Verification items for the finished model (mm, model axes). A direction names the side the tool comes from. Coordinates: 2 decimals unless noted, no trailing zeros. Order: outer loops, then holes, each group sorted by start corner. A loop starts at its lowest first (then second) coordinate and runs counter-clockwise, first axis right, second up. Notation, with made-up numbers: (-16.75, 11.25) -> (-5.75, 11.25) arc R20 cw to (-5.75, 37.25) -> close; hole circle Ø8 at (54.5, -6.75). An arc over 180 degrees is marked (long way). Answer as CSV lines item,"result".
```python
from build123d import *

# Parameters (mm, degrees)
SKETCH1_R           = 62.5
SKETCH1_R_2         = 22.5
BOSS_EXTRUDE1_DEPTH = 75
BOSS_EXTRUDE2_DEPTH = 25
SKETCH4_W           = 250
SKETCH4_H           = 270
BOSS_EXTRUDE3_DEPTH = 40
RIB5_REACH          = 417.482
SKETCH6_WALL_W      = 1103.483628374
SKETCH6_WALL_H      = 25
SKETCH9_R           = 6.25
SKETCH9_R_2         = 12.5
CUT_EXTRUDE4_DEPTH  = 40


with BuildPart() as part:
    # Sketch1 → Boss-Extrude1 (new body)
    with BuildSketch(Plane.XY):
        Circle(SKETCH1_R)
        Circle(SKETCH1_R_2, mode=Mode.SUBTRACT)
    extrude(amount=BOSS_EXTRUDE1_DEPTH)

    # Sketch3 → Boss-Extrude2 (add)
    with BuildSketch(Plane(origin=(0, 0, 0), x_dir=(-1, 0, 0), z_dir=(0, 0, -1))):
        with BuildLine():
            Line((-62.5, 0), (-125, -250))
            Line((-125, -250), (125, -250))
            Line((125, -250), (62.5, 0))
            ThreePointArc((62.5, 0), (0, -62.5), (-62.5, 0))
        make_face()
    extrude(amount=-BOSS_EXTRUDE2_DEPTH)

    # Sketch4 → Boss-Extrude3 (add)
    with BuildSketch(Plane.XZ.offset(250)):
        with Locations((0, 135)):
            Rectangle(SKETCH4_W, SKETCH4_H)
    extrude(amount=BOSS_EXTRUDE3_DEPTH)

    # Sketch6 wall → Rib5 (add, up to next)
    with BuildSketch(Plane(origin=(0, -156.25, 172.5), x_dir=(0, 0.693108716252, -0.720833064902), z_dir=(0, 0.720833064902, 0.693108716252)), mode=Mode.PRIVATE) as rib5_sk1:
        Rectangle(SKETCH6_WALL_W, SKETCH6_WALL_H)
    rib5_tool1 = extrude(rib5_sk1.sketch, amount=-RIB5_REACH, mode=Mode.PRIVATE) - part.part
    add(rib5_tool1.solids().sort_by_distance((0, -156.25, 172.5))[0])

    # Sketch9 → Cut-Extrude4 (cut)
    with BuildSketch(Plane.XZ.offset(290)):
        with Locations(Location((-110, 225, 0), (0, 0, 270))):
            Circle(SKETCH9_R)
        with Locations(Location((-110, 255, 0), (0, 0, 270))):
            Circle(SKETCH9_R)
        with Locations(Location((95, 75, 0), (0, 0, 270))):
            Circle(SKETCH9_R_2)
        with Locations(Location((-95, 240, 0), (0, 0, 270))):
            Circle(SKETCH9_R_2)
        with Locations(Location((-80, 255, 0), (0, 0, 270))):
            Circle(SKETCH9_R)
        with Locations(Location((-80, 225, 0), (0, 0, 270))):
            Circle(SKETCH9_R)
        with Locations(Location((110, 225, 0), (0, 0, 270))):
            Circle(SKETCH9_R)
        with Locations(Location((95, 240, 0), (0, 0, 270))):
            Circle(SKETCH9_R_2)
        with Locations(Location((110, 255, 0), (0, 0, 270))):
            Circle(SKETCH9_R)
        with Locations(Location((80, 255, 0), (0, 0, 270))):
            Circle(SKETCH9_R)
        with Locations(Location((80, 225, 0), (0, 0, 270))):
            Circle(SKETCH9_R)
        with Locations(Location((110, 90, 0), (0, 0, 270))):
            Circle(SKETCH9_R)
        with Locations(Location((110, 60, 0), (0, 0, 270))):
            Circle(SKETCH9_R)
        with Locations(Location((80, 60, 0), (0, 0, 270))):
            Circle(SKETCH9_R)
        with Locations(Location((80, 90, 0), (0, 0, 270))):
            Circle(SKETCH9_R)
        with Locations(Location((-80, 60, 0), (0, 0, 270))):
            Circle(SKETCH9_R)
        with Locations(Location((-80, 90, 0), (0, 0, 270))):
            Circle(SKETCH9_R)
        with Locations(Location((-110, 90, 0), (0, 0, 270))):
            Circle(SKETCH9_R)
        with Locations(Location((-110, 60, 0), (0, 0, 270))):
            Circle(SKETCH9_R)
        with Locations(Location((-95, 75, 0), (0, 0, 270))):
            Circle(SKETCH9_R_2)
    extrude(amount=-CUT_EXTRUDE4_DEPTH, mode=Mode.SUBTRACT)


solid = part.part
```
Item 1: Section check D-D, the plane z = 240. Record the boundary of the cut face in (x, y).
Answer list:
outline,"(-125, -290) -> (-107.5, -290) -> (-107.5, -250) -> (-125, -250) -> close; (-82.5, -290) -> (82.5, -290) -> (82.5, -250) -> (12.5, -250) -> (12.5, -221.15) -> (-12.5, -221.15) -> (-12.5, -250) -> (-82.5, -250) -> close; (107.5, -290) -> (125, -290) -> (125, -250) -> (107.5, -250) -> close"
Item 2: Section check B-B, the plane z = 47. Record the boundary of the cut face in (x, y), plus the area to 3 significant figures.
Answer list:
outline,"(-125, -290) -> (125, -290) -> (125, -250) -> (12.5, -250) -> (12.5, -61.24) arc R62.5 ccw (long way) to (-12.5, -61.24) -> (-12.5, -250) -> (-125, -250) -> close; hole circle Ø45 at (0, 0)"
area,"25,400 mm2"
Item 3: Depth check by flat-ended pin: pin 1 Ø14.5 at (x, z) = (-80, 225) entering from -Y; pin 2 Ø10 at (x, z) = (-46, 233.5) entering from +Y; pin 3 Ø8 at (y, z) = (-159, 70) entering from -X; pin 4 Ø1.5 at (y, z) = (-197, 114) entering from +X. Enter the tip coordinate at first touch or a pass-through.
Answer list:
pin 1,"y = -290"
pin 2,"y = -250"
pin 3,"x = -12.5"
pin 4,"x = 12.5"
Item 4: Tool access check on faces 1 (the cylindrical face through (114.22, -270.28, 229.61)), 2 (the flat face through (57, -151, 25)), 3 (the flat face through (-12.5, -192, 116)). Record the directions out of +Z, -Z, +X, -X, +Y, -Y that give a thin tool (end or side, any length) a straight path to the whole face; none if there is none.
Answer list:
face 1,"+Y, -Y"
face 2,"+Z, +X"
face 3,"+Z, -X"
Item 5: Section check C-C, the plane y = -146. Record the boundary of the cut face in (x, z).
Answer list:
outline,"(-99, 0) -> (99, 0) -> (99, 25) -> (12.5, 25) -> (12.5, 161.84) -> (-12.5, 161.84) -> (-12.5, 25) -> (-99, 25) -> close"
Item 6: Release check for a two-part mould opening along Z. For faces 4 (the cylindrical face through (-82.606, -270.28, 76.627)), 5 (the flat face through (-94.188, -126.75, 12.325)), 6 (the flat face through (-2, -150, 0)) record: +Z half, -Z half, draft (parallel to the pull), parting line (faces both ways), or undercut.
Answer list:
face 4,"undercut"
face 5,"draft"
face 6,"-Z half"
Item 7: Section check A-A, the plane x = 95. Record the boundary of the cut face in (y, z), plus the area to 3 significant figures.
Answer list:
outline,"(-290, 0) -> (-130, 0) -> (-130, 25) -> (-250, 25) -> (-250, 62.5) -> (-290, 62.5) -> close; (-290, 87.5) -> (-250, 87.5) -> (-250, 227.5) -> (-290, 227.5) -> close; (-290, 252.5) -> (-250, 252.5) -> (-250, 270) -> (-290, 270) -> close"
area,"11,800 mm2"
Item 8: Thickness scan on line 1 (X direction, y = -275, z = 255); line 2 (X direction, y = -281.5, z = 75); line 3 (Y direction, x = -114, z = 119). Record the ranges inside material, lowest first.
Answer list:
line 1,"-125 to -116.25, -103.75 to -86.25, -73.75 to 73.75, 86.25 to 103.75, 116.25 to 125"
line 2,"-125 to -107.5, -82.5 to 82.5, 107.5 to 125"
line 3,"-290 to -250"
